```python
from build123d import *

# Parameters (mm, degrees)
SKETCH1_R           = 30
SKETCH1_R_2         = 7.5
BOSS_EXTRUDE1_DEPTH = 15


with BuildPart() as part:
    # Sketch1 → Boss-Extrude1 (new body)
    with BuildSketch(Plane.XY):
        Circle(SKETCH1_R)
        Circle(SKETCH1_R_2, mode=Mode.SUBTRACT)
    extrude(amount=BOSS_EXTRUDE1_DEPTH)

    # Sketch2 → Revolve4 (revolve)
    with BuildSketch(Plane(origin=(0, 0, 0), x_dir=(1, 0, 0), z_dir=(0, 1, 0))):
        Polygon((7.5, 0), (30, 0), (39.62, 9.62), (25.477864376, 23.762135624), (17.967751926, 17), (7.5, 17), align=None)
    revolve(axis=Axis((0, 0, 0), (0, 0, -1)))


solid = part.part
```
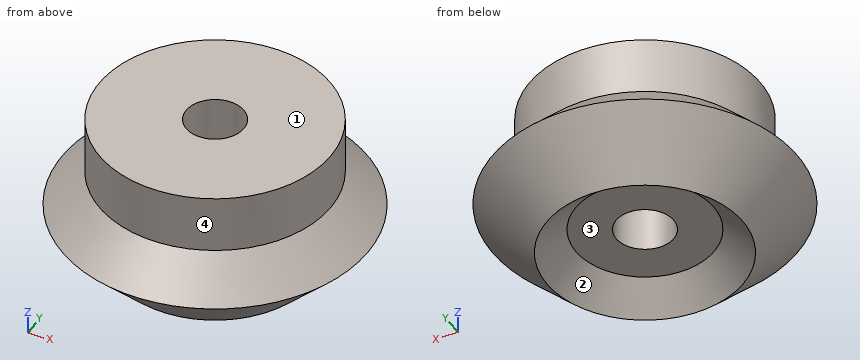
Work out the finished part from the listing and answer in its coordinate system (mm). Face numbers are marked on the shaded views. Give positions to 0.01 mm unless a question says otherwise; leave off trailing zeros. Loops run counter-clockwise (first coordinate to the right, second up) from the corner with the lowest first, then second, coordinate; pieces in that order, holes last. Notation, with made-up numbers: (-21.5, 72) -> (18.5, 72) arc R34 cw to (18.5, 105) -> close; hole circle Ø7 at (32.25, 10.5). An arc over 180 degrees is marked (long way). Put each result on its own line as item: value. Start each with the question number.
Item 1: The part is cut by section D-D (z = 12). Give the vertices of the cut face in (x, y).
Item 2: Each of these flat-tipped pins is pushed along its axis until it touches: P1, Ø9, axis at x = 0, y = 0, coming from the -Z side; P2, Ø1.5, axis at y = -23, z = -9.5, coming from the +X side; P3, Ø12, axis at y = -21, z = -2.5, coming from the -X side; P4, Ø6, axis at x = 22, z = -2.5, coming from the -Y side. Where does it stop, or does it pass through?
Item 3: The part is cut by section A-A (x = 0). Give the vertices of the cut face in (y, z).
Item 4: The part is cut by section C-C (z = -12). Give the vertices of the cut face in (x, y).
Item 5: Find the intervals of material crossed by L1, parallel to Y at x = 0, z = 7; L2, parallel to Y at x = 0, z = -8; L3, parallel to X at y = 0, z = -9, in increasing order. Write a range as [from, to].
Item 6: The mould has two halves that part along Y. Classify the marked faces 1, 2, 3 and 4: released by +Y, released by -Y, zero draft, split by the parting line, or undercut.
Answers below:
1. outline: circle Ø60 at (0, 0); hole circle Ø15 at (0, 0)
2. P1: through
2. P2: x = 32.78
2. P3: x = -33.14
2. P4: y = -28.49
3. outline: (-39.62, -9.62) -> (-25.48, -23.76) -> (-17.97, -17) -> (-7.5, -17) -> (-7.5, 15) -> (-30, 15) -> (-30, 0) -> close; (7.5, -17) -> (17.97, -17) -> (25.48, -23.76) -> (39.62, -9.62) -> (30, 0) -> (30, 15) -> (7.5, 15) -> close
4. outline: circle Ø74.48 at (0, 0); hole circle Ø15 at (0, 0)
5. L1: [-30, -7.5], [7.5, 30]
5. L2: [-38, -7.5], [7.5, 38]
5. L3: [-39, -7.5], [7.5, 39]
6. face 1: zero draft
6. face 2: undercut
6. face 3: undercut
6. face 4: split by the parting line
